Check sheet for the modelled part. Datum: model origin and axes. Units: mm. Face numbers are marked on the shaded views. Round coordinates to 2 decimals unless told otherwise and drop trailing zeros. Write each loop counter-clockwise with the first axis right and the second up, starting at its lowest first coordinate (ties: lowest second). Pieces come first, ordered by that corner, then holes.
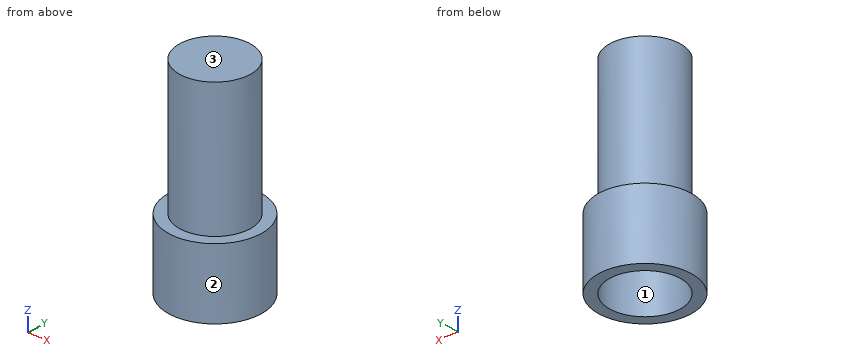
from build123d import *

# Parameters (mm, degrees)
F0_R     = 5.25
F0_R_2   = 4
F1_DEPTH = 7.8
F2_DEPTH = 5
F3_R     = 4
F4_DEPTH = 15


with BuildPart() as f1:
    # F0 (on Top) → F1 (new body)
    with BuildSketch(Plane.XY):
        Circle(F0_R)
        Circle(F0_R_2, mode=Mode.SUBTRACT)
        Circle(F0_R_2)
    extrude(amount=F1_DEPTH)

    # F0 (on Top) → F2 (cut)
    with BuildSketch(Plane.XY):
        Circle(F0_R_2)
    extrude(amount=F2_DEPTH, mode=Mode.SUBTRACT)

    # F3 (on face) → F4 (join)
    with BuildSketch(Plane.XY.offset(7.8)):
        Circle(F3_R)
    extrude(amount=F4_DEPTH)


solid = f1.part
1. Sectioned sample at A-A, the plane x = 0. Enter the section's corners in (y, z), plus the area to 3 significant figures.
2. Go/stop test with flat-tipped pins: pin 1 (6 mm diameter, centred on y = -0.5, z = 11, fed in from +X); pin 2 (1 mm diameter, centred on y = -1, z = 17, fed in from -X); pin 3 (1 mm diameter, centred on x = 4, z = 2.5, fed in from +Y). Record where each tip stops, or that it passes through.
3. Sectioned sample at C-C, the plane z = 19.5. Enter the section's corners in (x, y), plus the area to 3 significant figures.
4. Release check for a two-part mould opening along Y. For the marked faces 1, 2 and 3 record: released by +Y, released by -Y, zero draft, split by the parting line, or undercut.
5. Scan lines: line 1 along Y through (x, z) = (0, 2.95); line 2 along Z through (x, y) = (0, -3.5); line 3 along X through (y, z) = (3.5, 2.5). Record each from-to range of solid material in increasing order.
6. Sectioned sample at D-D, the plane y = -4.5. Enter the section's corners in (x, z).
Computed values:
1. outline: (-5.25, 0) - (-4, 0) - (-4, 5) - (4, 5) - (4, 0) - (5.25, 0) - (5.25, 7.8) - (4, 7.8) - (4, 22.8) - (-4, 22.8) - (-4, 7.8) - (-5.25, 7.8) - close
1. area: 162 mm2
2. pin 1: stops at x = 4
2. pin 2: stops at x = -3.97
2. pin 3: stops at y = 3.91
3. outline: circle Ø8 at (0, 0)
3. area: 50.3 mm2
4. face 1: undercut
4. face 2: split by the parting line
4. face 3: zero draft
5. line 1: y = -5.25 to -4, 4 to 5.25
5. line 2: z = 5 to 22.8
5. line 3: x = -3.91 to -1.94, 1.94 to 3.91
6. outline: (-2.7, 0) - (2.7, 0) - (2.7, 7.8) - (-2.7, 7.8) - close
